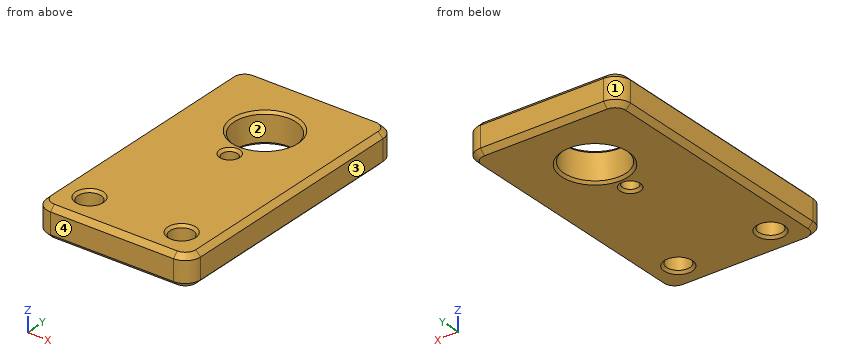
```python
from build123d import *

# Parameters (mm, degrees)
SKETCH1_W                       = 15.875
SKETCH1_H                       = 27.78125
BOSS_EXTRUDE1_DEPTH             = 1.5875
F_3_32_0_09375_DIAMETER_HOLE1_D = 2.38125
F_1_4_0_25_DIAMETER_HOLE1_D     = 6.35
F_1_16_0_0625_DIAMETER_HOLE1_D  = 1.5875
FILLET1_R                       = 1.5875
CHAMFER1_SIZE                   = 0.508
CHAMFER2_SIZE                   = 0.254


with BuildPart() as part:
    # Sketch1 → Boss-Extrude1 (new body, symmetric)
    with BuildSketch(Plane.XY):
        Rectangle(SKETCH1_W, SKETCH1_H)
    extrude(amount=BOSS_EXTRUDE1_DEPTH, both=True)

    # 3/32 (0.09375) Diameter Hole1 (through all)
    with Locations(Plane.XY.offset(1.5875)):
        with Locations((-4.7625, -10.715625), (4.7625, -10.715625)):
            Hole(F_3_32_0_09375_DIAMETER_HOLE1_D / 2)

    # 1/4 (0.25) Diameter Hole1 (through all)
    with Locations(Plane.XY.offset(1.5875)):
        with Locations((0, 6.746875)):
            Hole(F_1_4_0_25_DIAMETER_HOLE1_D / 2)

    # 1/16 (0.0625) Diameter Hole1 (through all)
    with Locations(Plane.XY.offset(1.5875)):
        with Locations((0, 1.984375)):
            Hole(F_1_16_0_0625_DIAMETER_HOLE1_D / 2)

    # Fillet1
    fillet1_edges = [part.edges().sort_by_distance(p)[0] for p in [
        (-7.9375, -13.890625, 0),
        (7.9375, -13.890625, 0),
        (7.9375, 13.890625, 0),
        (-7.9375, 13.890625, 0),
    ]]
    fillet(fillet1_edges, radius=FILLET1_R)

    # Chamfer1
    chamfer1_edges = [part.edges().sort_by_distance(p)[0] for p in [
        (7.9375, 0, -1.5875),
        (7.9375, 0, 1.5875),
        (-7.9375, 0, -1.5875),
        (0, 13.890625, -1.5875),
        (0, -13.890625, -1.5875),
        (7.472532015, 13.425657015, -1.5875),
        (-7.472532015, 13.425657015, -1.5875),
        (-7.472532015, -13.425657015, -1.5875),
        (7.472532015, -13.425657015, -1.5875),
        (0, -13.890625, 1.5875),
        (-7.9375, 0, 1.5875),
        (0, 13.890625, 1.5875),
        (7.472532015, 13.425657015, 1.5875),
        (-7.472532015, 13.425657015, 1.5875),
        (-7.472532015, -13.425657015, 1.5875),
        (7.472532015, -13.425657015, 1.5875),
    ]]
    chamfer(chamfer1_edges, length=CHAMFER1_SIZE)

    # Chamfer2
    chamfer2_edges = [part.edges().sort_by_distance(p)[0] for p in [
        (5.953125, -10.715625, 1.5875),
        (5.953125, -10.715625, -1.5875),
        (-3.571875, -10.715625, 1.5875),
        (-3.571875, -10.715625, -1.5875),
        (3.175, 6.746875, 1.5875),
        (3.175, 6.746875, -1.5875),
        (0.79375, 1.984375, 1.5875),
        (0.79375, 1.984375, -1.5875),
    ]]
    chamfer(chamfer2_edges, length=CHAMFER2_SIZE)


solid = part.part
```
Input: part model. Units: mm. Frame: model coordinates. Face numbers are marked on the shaded views. Give positions to 0.01 mm unless a question says otherwise; leave off trailing zeros. Order: outer loops, then holes, each group sorted by start corner. A loop starts at its lowest first (then second) coordinate and runs counter-clockwise, first axis right, second up. Notation, with made-up numbers: (-24.75, 49.5) - (-17.75, 49.5) arc R35 cw to (-17.75, 82.5) - close; hole circle Ø2 at (5.5, 46.5). An arc over 180 degrees is marked (long way). Use a Markdown table: item, result.
(1) Pin query (flat end, axial travel): pin 1 (1.3 mm diameter, centred on x = 0, y = 1.98, fed in from +Z); pin 2 (1.5 mm diameter, centred on x = -2.5, y = 6.5, fed in from +Z). Return the tip coordinate at first contact, or that it passes through.
Computed values:
| item | result |
|---|---|
| pin 1 | passes through |
| pin 2 | stops at z = 1.42 |
(2) Section query A-A (x = 0). Output: boundary loops of the cut face in (y, z).
Computed values:
| item | result |
|---|---|
| outline | (-13.89, -1.08) - (-13.38, -1.59) - (0.94, -1.59) - (1.19, -1.33) - (1.19, 1.33) - (0.94, 1.59) - (-13.38, 1.59) - (-13.89, 1.08) - close; (2.78, -1.33) - (3.03, -1.59) - (3.32, -1.59) - (3.57, -1.33) - (3.57, 1.33) - (3.32, 1.59) - (3.03, 1.59) - (2.78, 1.33) - close; (9.92, -1.33) - (10.18, -1.59) - (13.38, -1.59) - (13.89, -1.08) - (13.89, 1.08) - (13.38, 1.59) - (10.18, 1.59) - (9.92, 1.33) - close |
(3) Draft query along Y for the marked faces 1, 2, 3 and 4. Return one class per face: released by +Y, released by -Y, zero draft, split by the parting line, or undercut.
Computed values:
| item | result |
|---|---|
| face 1 | released by +Y |
| face 2 | undercut |
| face 3 | zero draft |
| face 4 | released by -Y |
(4) Section query B-B (z = -0.7). State how many separate pieces and enclosed holes the cut face has, then the cut area to 3 significant figures.
Computed values:
| item | result |
|---|---|
| separate pieces | 1 |
| enclosed holes | 4 |
| area | 396 mm2 |
(5) Line query: line 1 (Y direction, x = 0, z = -0.2); line 2 (Y direction, x = 2.75, z = -1.35); line 3 (X direction, y = 5.75, z = 1.1). Output: solid intervals per line, ascending. Write a range as from..to.
Computed values:
| item | result |
|---|---|
| line 1 | y = -13.89..1.19, 2.78..3.57, 9.92..13.89 |
| line 2 | y = -13.62..5.13, 8.37..13.62 |
| line 3 | x = -7.92..-3.01, 3.01..7.92 |
